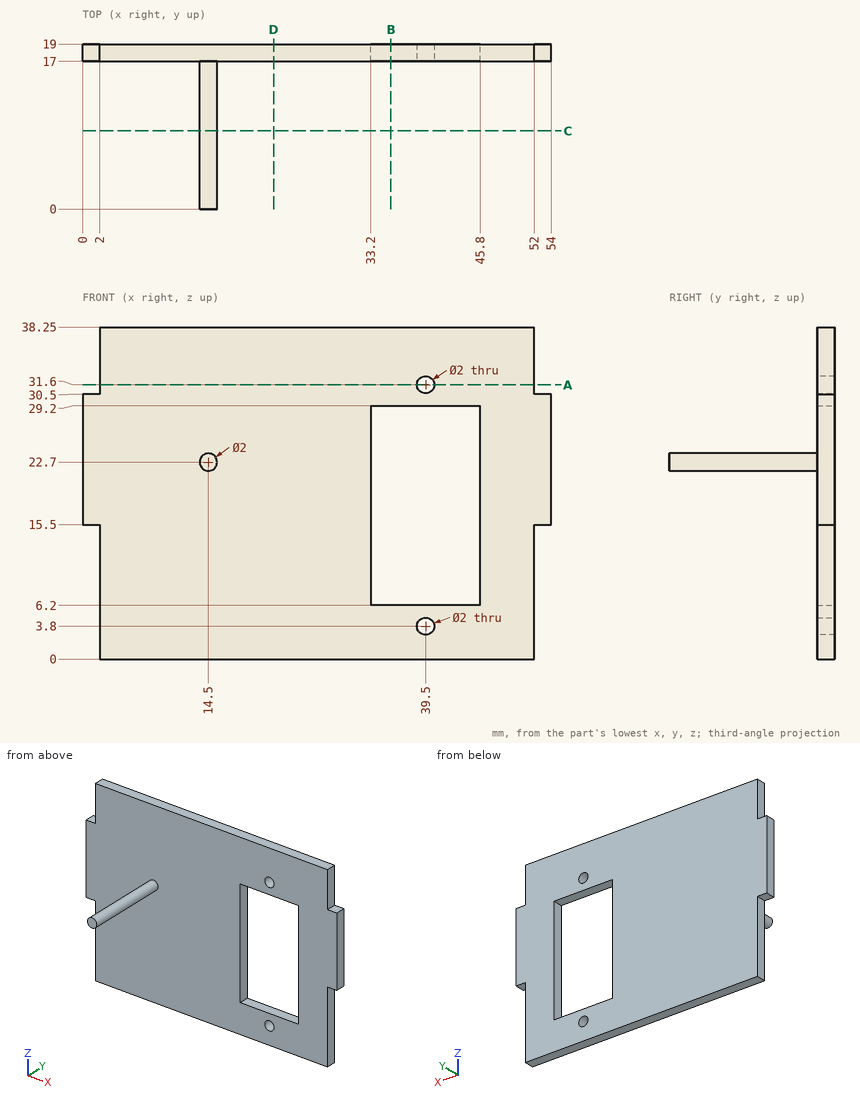
Check sheet for the drawn part. Datum: minimum x, y, z corner. Units: mm. Round coordinates to 2 decimals unless told otherwise and drop trailing zeros. Loops run counter-clockwise (first coordinate to the right, second up) from the corner with the lowest first, then second, coordinate; pieces in that order, holes last. Notation, with made-up numbers: (-0.5, -2) - (41.5, -2) arc R15 cw to (41.5, 23) - close; hole circle Ø2 at (-13, -18). An arc over 180 degrees is marked (long way). Write each question's results on one line, items separated by ' | '. Start each with the question number.
Q1. Cross-section at D-D on x = 22. Enter the section's corners in (y, z).
Q2. Cross-section at B-B on x = 35.5. Enter the section's corners in (y, z), and give its area (3 significant figures).
Q3. Cross-section at A-A on z = 31.6. Enter the section's corners in (x, y).
Q4. Cross-section at C-C on y = 9. Enter the section's corners in (x, z).
Q5. Thickness scan on line 1 (Z direction, x = 39.5, y = 18.6); line 2 (X direction, y = 17.55, z = 31.6); line 3 (Y direction, x = 19.5, z = 19). Record the ranges inside material, lowest first. Write a range as [from, to].
Q6. Gauge pin test, flat ends, axial feed: P1, Ø0.6, axis at y = 18, z = 35.5, coming from the -X side; P2, Ø1, axis at x = 0.5, y = 18, coming from the +Z side; P3, Ø6, axis at x = 46, y = 15.5, coming from the +Z side; P4, Ø0.6, axis at x = 53, y = 17.5, coming from the -Z side. Record the tip position at first contact, or that the pin passes through.
Answers below:
1) outline: (17, 0) - (19, 0) - (19, 38.25) - (17, 38.25) - close
2) outline: (17, 0) - (19, 0) - (19, 6.2) - (17, 6.2) - close; (17, 29.2) - (19, 29.2) - (19, 38.25) - (17, 38.25) - close | area: 30.5 mm²
3) outline: (2, 17) - (38.5, 17) - (38.5, 19) - (2, 19) - close; (40.5, 17) - (52, 17) - (52, 19) - (40.5, 19) - close
4) outline: circle Ø2 at (14.5, 22.7)
5) line 1: z = [0, 2.8], [4.8, 6.2], [29.2, 30.6], [32.6, 38.25] | line 2: x = [2, 38.5], [40.5, 52] | line 3: y = [17, 19]
6) P1: stops at x = 2 | P2: stops at z = 30.5 | P3: stops at z = 38.25 | P4: stops at z = 15.5
